Could you check a few things on this model? Use its own coordinates, in mm. A direction names the side the tool comes from. Give positions to 0.01 mm unless a question says otherwise; leave off trailing zeros. Loops run counter-clockwise (first coordinate to the right, second up) from the corner with the lowest first, then second, coordinate; pieces in that order, holes last. Notation, with made-up numbers: (7, 0) - (39, 0) arc R26 ccw to (39, 28) - close; hole circle Ø9 at (-24.75, 77). An arc over 180 degrees is marked (long way). One line per item, written item: value. Start each with the question number.
Q1. I want a section at C-C (x = -18). Please give me the cut outline in (y, z).
Q2. I'm going to push flat-ended pins straight in: P1, Ø9.5, axis at x = 0, y = 0, coming from the -Z side; P2, Ø1.5, axis at x = -1, z = 0, coming from the +Y side; P3, Ø2, axis at y = 24, z = -3, coming from the -X side. Where does each tip first touch, or does it pass through?
Q3. I want a section at A-A (y = 0). Please give me the cut outline in (x, z), then the cut area to 3 significant figures.
Q4. I want a section at D-D (x = 9). Please give me the cut outline in (y, z), then the cut area to 3 significant figures.
Q5. I want a section at B-B (z = -0.25). Please give me the cut outline in (x, y).
Q6. For faces 4 (the face through (-7, 10, 2.5)), 5 (the face through (-26, -8, 0)), 6 (the face through (-17.814, 25.56, 0.035)), which set-ups out of +Z, -Z, +X, -X, +Y, -Y let a thin tool reach every point of the face, with its end or its side?
Q7. If I drill on line 1 (Z direction, x = -31.5, y = 5); line 2 (Y direction, x = 0, z = 0.25); line 3 (X direction, y = -1, z = 2), over which ranges is the centre line in solid material (lowest first)? Write a range as from..to.
Q8. If we mould it in two halves opening along Y, with no side actions, what happens to faces 1 (the face through (-10, 0, -3)), 2 (the face through (-26, 8, 0)), 3 (the face through (-6.63, 29.94, 0.04))? For each: released by +Y, released by -Y, zero draft, split by the parting line, or undercut.
```python
from build123d import *

# Parameters (mm, degrees)
BOSS_EXTRU_1_DEPTH      = 2.5
ESQUISSE2_R             = 10
BOSS_EXTRU_2_DEPTH      = 1.25
ESQUISSE3_R             = 6
ENL_V_MAT_EXTRU_1_DEPTH = 62.539171077


with BuildPart() as part:
    # Esquisse1 → Boss.-Extru.1 (new, symmetric)
    with BuildSketch(Plane.XY):
        with BuildLine():
            Line((0.392596459, 13.994494204), (-10.5894536, 9.157700172))
            ThreePointArc((-10.5894536, 9.157700172), (-11.054455161, 8.590635663), (-11.489125293, 8))
            Line((-11.489125293, 8), (-11.489125293, -8))
            ThreePointArc((-11.489125293, -8), (4.192388692, -13.357540082), (14, 0))
            ThreePointArc((14, 0), (10.03733905, 9.759704134), (0.392596459, 13.994494204))
        make_face()
        with BuildLine():
            ThreePointArc((0.392596459, 13.994494204), (-5.64292637, 12.812391735), (-10.5894536, 9.157700172))
            Line((-10.5894536, 9.157700172), (0.392596459, 13.994494204))
        make_face()
        with BuildLine():
            Line((-11.489125293, -8), (-11.489125293, 8))
            ThreePointArc((-11.489125293, 8), (-14, 0), (-11.489125293, -8))
        make_face()
        with BuildLine():
            ThreePointArc((-11.489125293, -8), (-14, 0), (-11.489125293, 8))
            Line((-11.489125293, 8), (-40, 8))
            Line((-40, 8), (-40, -8))
            Line((-40, -8), (-11.489125293, -8))
        make_face()
        with BuildLine():
            Line((-13.856151097, 46.346597251), (-24.838201156, 41.50980322))
            Line((-24.838201156, 41.50980322), (-10.5894536, 9.157700172))
            ThreePointArc((-10.5894536, 9.157700172), (-5.64292637, 12.812391735), (0.392596459, 13.994494204))
            Line((0.392596459, 13.994494204), (-13.856151097, 46.346597251))
        make_face()
    extrude(amount=BOSS_EXTRU_1_DEPTH, both=True)

    # Esquisse2 → Boss.-Extru.2 (add, symmetric)
    with BuildSketch(Plane(origin=(0, 0, -2.5), x_dir=(-1, 0, 0), z_dir=(0, 0, -1))):
        with Locations(Location((0, 0, 0), (0, 0, 180))):
            Circle(ESQUISSE2_R)
    extrude(amount=BOSS_EXTRU_2_DEPTH, both=True)

    # Esquisse3 → Enlèv. mat.-Extru.1 (cut, through all)
    with BuildSketch(Plane(origin=(0, 0, -3.75), x_dir=(-1, 0, 0), z_dir=(0, 0, -1))):
        Circle(ESQUISSE3_R)
    extrude(amount=-ENL_V_MAT_EXTRU_1_DEPTH, mode=Mode.SUBTRACT)


solid = part.part
```
Worked answers:
1. outline: (-8, -2.5) - (8, -2.5) - (8, 2.5) - (-8, 2.5) - close; (25.98, -2.5) - (44.52, -2.5) - (44.52, 2.5) - (25.98, 2.5) - close
2. P1: passes through
2. P2: stops at y = 18.86
2. P3: stops at x = -17.51
3. outline: (-40, -2.5) - (-10, -2.5) - (-10, -3.75) - (-6, -3.75) - (-6, 2.5) - (-40, 2.5) - close; (6, -3.75) - (10, -3.75) - (10, -2.5) - (14, -2.5) - (14, 2.5) - (6, 2.5) - close
3. area: 220 mm²
4. outline: (-10.72, -2.5) - (-4.36, -2.5) - (-4.36, -3.75) - (4.36, -3.75) - (4.36, -2.5) - (10.72, -2.5) - (10.72, 2.5) - (-10.72, 2.5) - close
4. area: 118 mm²
5. outline: (-40, -8) - (-11.49, -8) arc R14 ccw (long way) to (0.39, 13.99) - (-13.86, 46.35) - (-24.84, 41.51) - (-10.59, 9.16) arc R14 ccw to (-11.49, 8) - (-40, 8) - close; hole circle Ø12 at (0, 0)
6. face 4: +Z, +X, -X, +Y, -Y
6. face 5: +Z, -Z, -X, -Y
6. face 6: +Z, -Z, -X
7. line 1: z = -2.5..2.5
7. line 2: y = -14..-6, 6..14.89
7. line 3: x = -40..-5.92, 5.92..13.96
8. face 1: split by the parting line
8. face 2: undercut
8. face 3: released by +Y
